Check sheet for the modelled part. Datum: model origin and axes. Units: mm. Face numbers are marked on the shaded views. Give positions to 0.01 mm unless a question says otherwise; leave off trailing zeros. Order: outer loops, then holes, each group sorted by start corner. A loop starts at its lowest first (then second) coordinate and runs counter-clockwise, first axis right, second up.
```python
from build123d import *

# Parameters (mm, degrees)
SKETCH007_W     = 1
SKETCH007_H     = 15
PAD002_DEPTH    = 10
ARRAY_COUNT     = 6
SKETCH005_R     = 6.5
SKETCH004_R     = 4.5
SKETCH003_R     = 5.5
SKETCH002_R     = 6.5
SKETCH_R        = 6
PAD_DEPTH       = 1.75
SKETCH001_R     = 5.5
PAD001_DEPTH    = 3.5
SKETCH006_R     = 4.5
POCKET_DEPTH    = 8.751
CHAMFER_SIZE    = 1
SKETCH008_W     = 3.25
SKETCH008_H     = 1.5
POCKET001_DEPTH = 20.001
SKETCH009_W     = 3.25
SKETCH009_H     = 10
POCKET002_DEPTH = 1


with BuildPart() as array:
    # Sketch007 → Pad002 (new body)
    with BuildSketch(Plane.XY.offset(2)):
        with Locations((25.113381, 7.5)):
            Rectangle(SKETCH007_W, SKETCH007_H)
    extrude(amount=PAD002_DEPTH)

    # Array: Array ×6 about axis
    array_axis = Axis((25, 0, 0), (0, 0, 1))


with BuildPart() as array_1:
    add(array.part)
    for i in range(1, ARRAY_COUNT):
        add(array.part.rotate(array_axis, i * 360 / ARRAY_COUNT))


with BuildPart() as loft001:
    # Sketch005 → Loft001 section 0
    with BuildSketch(Plane.XY.offset(6)):
        with Locations((25, 0)):
            Circle(SKETCH005_R)
    # Sketch004 → Loft001 section 1
    with BuildSketch(Plane.XY.offset(7)):
        with Locations((25, 0)):
            Circle(SKETCH004_R)
    loft(ruled=True)


with BuildPart() as loft_body:
    # Sketch003 → Loft section 0
    with BuildSketch(Plane.XY.offset(5.25)):
        with Locations((25, 0)):
            Circle(SKETCH003_R)
    # Sketch002 → Loft section 1
    with BuildSketch(Plane.XY.offset(6)):
        with Locations((25, 0)):
            Circle(SKETCH002_R)
    loft(ruled=True)


with BuildPart() as pocket002:
    # Sketch → Pad (new body, symmetric)
    with BuildSketch(Plane.XY):
        with BuildLine():
            ThreePointArc((-25, 10), (-35, 0), (-25, -10))
            Line((-25, -10), (25, -10))
            ThreePointArc((25, -10), (35, 0), (25, 10))
            Line((-25, 10), (25, 10))
        make_face()
        with Locations((-25, 0)):
            Circle(SKETCH_R, mode=Mode.SUBTRACT)
    extrude(amount=PAD_DEPTH, both=True)

    # Sketch001 → Pad001 (new body)
    with BuildSketch(Plane.XY.offset(1.75)):
        with Locations((25, 0)):
            Circle(SKETCH001_R)
    extrude(amount=PAD001_DEPTH)

    # Fusion: union Loft body
    add(loft_body.part)

    # Fusion001: union Loft001
    add(loft001.part)

    # Sketch006 → Pocket (cut, through all)
    with BuildSketch(Plane.XY.offset(7)):
        with Locations((25, 0)):
            Circle(SKETCH006_R)
    extrude(amount=-POCKET_DEPTH, mode=Mode.SUBTRACT)

    # Cut: cut Array
    add(array_1.part, mode=Mode.SUBTRACT)

    # Chamfer
    chamfer_edges = [pocket002.edges().sort_by_distance(p)[0] for p in [
        (-31, 0, 1.75),
        (-31, 0, -1.75),
    ]]
    chamfer(chamfer_edges, length=CHAMFER_SIZE)

    # Sketch008 → Pocket001 (cut, through all)
    with BuildSketch(Plane.XZ.offset(10)):
        with Locations((-11.625, 0)):
            Rectangle(SKETCH008_W, SKETCH008_H)
        with Locations((11.625, 0)):
            Rectangle(SKETCH008_W, SKETCH008_H)
    extrude(amount=-POCKET001_DEPTH, mode=Mode.SUBTRACT)

    # Sketch009 → Pocket002 (cut)
    with BuildSketch(Plane(origin=(0, 0, -1.75), x_dir=(1, 0, 0), z_dir=(0, 0, -1))):
        with Locations((-11.625, 7.5)):
            Rectangle(SKETCH009_W, SKETCH009_H)
        with Locations((-11.625, -7.5)):
            Rectangle(SKETCH009_W, SKETCH009_H)
        with Locations((11.625, 7.5)):
            Rectangle(SKETCH009_W, SKETCH009_H)
        with Locations((11.625, -7.5)):
            Rectangle(SKETCH009_W, SKETCH009_H)
    extrude(amount=-POCKET002_DEPTH, mode=Mode.SUBTRACT)


solid = pocket002.part
```
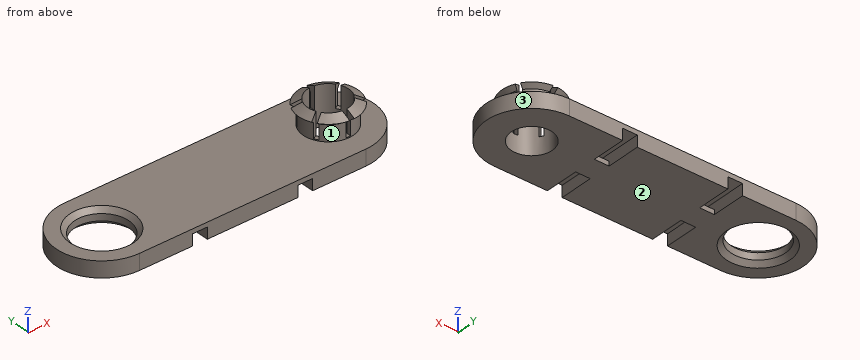
(1) Gauge pin test, flat ends, axial feed: pin 1 Ø0.6 at (y, z) = (5, 4) entering from +X; pin 2 Ø0.8 at (y, z) = (-4, -0.5) entering from +X; pin 3 Ø0.8 at (x, z) = (-12, -1) entering from -Y; pin 4 Ø5 at (x, z) = (4, 4.5) entering from +Y. Record the tip position at first contact, or that the pin passes through.
Response values:
pin 1: stops at x = 27.86
pin 2: stops at x = 34.33
pin 3: stops at y = -2.5
pin 4: passes through
(2) Cross-section at C-C on z = 3. Enter the section's corners in (x, y).
Response values:
outline: (19.96, -2.2) - (20.83, -1.7) arc R4.5 cw to (20.92, 1.91) - (20.06, 2.41) arc R5.5 ccw to start; (20.44, -3.08) arc R5.5 ccw to (24.39, -5.47) - (24.39, -4.46) arc R4.5 cw to (21.31, -2.58) - close; (20.57, 3.26) - (21.45, 2.76) arc R4.5 cw to (24.61, 4.48) - (24.61, 5.49) arc R5.5 ccw to start; (25.39, -5.49) arc R5.5 ccw to (29.43, -3.26) - (28.55, -2.76) arc R4.5 cw to (25.39, -4.48) - close; (25.61, 4.46) arc R4.5 cw to (28.69, 2.58) - (29.56, 3.08) arc R5.5 ccw to (25.61, 5.47) - close; (29.08, -1.91) - (29.94, -2.41) arc R5.5 ccw to (30.04, 2.2) - (29.17, 1.7) arc R4.5 cw to start
(3) Release check for a two-part mould opening along Z. For the marked faces 1, 2 and 3 record: released by +Z, released by -Z, zero draft, split by the parting line, or undercut.
Response values:
face 1: undercut
face 2: released by -Z
face 3: zero draft
(4) Material ranges on L1, parallel to Y at x = -25, z = 0.3; L2, parallel to X at y = -4, z = 0.5; L3, parallel to X at y = 0, z = 1, recorded low to high.
Response values:
L1: y = -10 to -6, 6 to 10
L2: x = -34.17 to -29.47, -20.53 to -13.25, -10 to 10, 13.25 to 22.94, 27.06 to 34.17
L3: x = -35 to -31.25, -18.75 to 20.5, 29.5 to 35
(5) Cross-section at B-B on y = -8. Enter the section's corners in (x, z).
Response values:
outline: (-31, -1.75) - (-13.25, -1.75) - (-13.25, 0.75) - (-10, 0.75) - (-10, -1.75) - (10, -1.75) - (10, 0.75) - (13.25, 0.75) - (13.25, -1.75) - (31, -1.75) - (31, 1.75) - (-31, 1.75) - close
(6) Cross-section at D-D on x = -16. Enter the section's corners in (y, z), then the cut area to 3 significant figures.
Response values:
outline: (-10, -1.75) - (10, -1.75) - (10, 1.75) - (-10, 1.75) - close
area: 70.0 mm2
(7) Cross-section at A-A on y = 0. Count the separate pieces of the cut face and the enclosed holes in it, then the cut area to 3 significant figures.
Response values:
separate pieces: 3
enclosed holes: 2
area: 171 mm2
